from build123d import *

# Parameters (mm, degrees)
F0_R     = 10
F1_DEPTH = 40
F2_W     = 65
F2_H     = 15
F3_DEPTH = 5
F4_R     = 7.5
F5_DEPTH = 30


with BuildPart() as f1:
    # F0 (on Front) → F1 (new body)
    with BuildSketch(Plane.XZ):
        Circle(F0_R)
    extrude(amount=F1_DEPTH)

    # F2 (on face) → F3 (join)
    with BuildSketch(Plane(origin=(0, 0, 0), x_dir=(-1, 0, 0), z_dir=(0, 1, 0))):
        Rectangle(F2_W, F2_H)
    extrude(amount=-F3_DEPTH)

    # F4 (on face) → F5 (join)
    with BuildSketch(Plane(origin=(0, 0, 0), x_dir=(-1, 0, 0), z_dir=(0, 1, 0))):
        Circle(F4_R)
        with Locations((-25, 0)):
            Circle(F4_R)
        with Locations((25, 0)):
            Circle(F4_R)
    extrude(amount=F5_DEPTH)


solid = f1.part
Model file for the job. Use its own axes, mm. A direction names the side the tool comes from. Round coordinates to 2 decimals unless told otherwise and drop trailing zeros. Order: outer loops, then holes, each group sorted by start corner. A loop starts at its lowest first (then second) coordinate and runs counter-clockwise, first axis right, second up. Notation, with made-up numbers: M 36.25,0.5 L 71.25,0.5 A28 ccw 71.25,33.5 Z; hole C 1.5,42.5 d4. An arc over 180 degrees is marked long. Write each question's results on one line, items separated by ' | '. Start each with the question number.
(1) Saw through at C-C, the plane z = -1. Give the cut face in (x, y).
(2) Saw through at B-B, the plane y = -4. Give the cut face in (x, z).
(3) Probe probe 1 along X at (y, z) = (18, -1); probe 2 along X at (y, z) = (23, 2.75); probe 3 along Y at (x, z) = (16.5, -3.5). List the from-to ranges inside material, lowest first. Write a range as from..to.
(4) Saw through at A-A, the plane x = 0. Give the cut face in (y, z).
(5) Drop flat-ended pins along their axis: pin 1 (4.5 mm diameter, centred on x = 17, z = -3, fed in from -Y); pin 2 (5.5 mm diameter, centred on x = 18, y = -3, fed in from +Z); pin 3 (2 mm diameter, centred on y = 10.5, z = 4.5, fed in from -X). Give the stop position or say it passes through.
(6) Which spindle directions (+Z, -Z, +X, -X, +Y, -Y) get a long thin tool onto all of the face, cutting with end or side? Do faces 1 (the face through (-31, 0, 6)), 2 (the face through (20, -2, 7.5)), 3 (the face through (-31, 0, -6)). Say none if no direction does.
(7) Two-plate mould, pull along X, no slides. Class faces 4 (the face through (-32.5, -2, 0)), 5 (the face through (7.493, 14.79, 0.33)), 6 (the face through (-19, -5, 0)): pulls with the +X half, pulls with the -X half, needs draft (parallel to the pull), parting line crosses it, or undercut.
(8) Saw through at D-D, the plane y = 4.5. Give the cut face in (x, z), then the cut area to 3 significant figures.
Established:
1) outline: M -32.5,-5 L -9.95,-5 L -9.95,-40 L 9.95,-40 L 9.95,-5 L 32.5,-5 L 32.5,0 L 32.43,0 L 32.43,30 L 17.57,30 L 17.57,0 L 7.43,0 L 7.43,30 L -7.43,30 L -7.43,0 L -17.57,0 L -17.57,30 L -32.43,30 L -32.43,0 L -32.5,0 Z
2) outline: M -32.5,-7.5 L -6.61,-7.5 A10 ccw 6.61,-7.5 L 32.5,-7.5 L 32.5,7.5 L 6.61,7.5 A10 ccw -6.61,7.5 L -32.5,7.5 Z
3) probe 1: x = -32.43..-17.57, -7.43..7.43, 17.57..32.43 | probe 2: x = -31.98..-18.02, -6.98..6.98, 18.02..31.98 | probe 3: y = -5..0
4) outline: M -40,-10 L 0,-10 L 0,-7.5 L 30,-7.5 L 30,7.5 L 0,7.5 L 0,10 L -40,10 Z
5) pin 1: stops at y = -5 | pin 2: stops at z = 7.5 | pin 3: stops at x = -31.63
6) face 1: +Z, -X, +Y | face 2: +Z, +X, +Y, -Y | face 3: -Z, -X, +Y
7) face 4: pulls with the -X half | face 5: undercut | face 6: needs draft
8) outline: C -25,0 d15; C 0,0 d15; C 25,0 d15 | area: 530 mm^2
